Can you work these out from the model? Positions are in its coordinate system, mm. A direction names the side the tool comes from. Give positions to 0.01 mm unless a question says otherwise; leave off trailing zeros. Loops run counter-clockwise (first coordinate to the right, second up) from the corner with the lowest first, then second, coordinate; pieces in that order, holes last. Notation, with made-up numbers: (-16, 28.5) -> (0, 28.5) arc R19 cw to (0, 64.5) -> close; hole circle Ø10 at (11.5, 73.5). An arc over 180 degrees is marked (long way). One line per question, with ' | ' between items.
from build123d import *

# Parameters (mm, degrees)
SKETCH1_W               = 117.475
SKETCH1_H               = 4.7625
BOSS_EXTRUDE1_DEPTH     = 50.8
F_1_2_HOLES_DEPTH       = 78.803697293
SKETCH7_W               = 170.933784369
SKETCH7_H               = 70.3072
BOSS_EXTRUDE2_DEPTH     = 164.9349
CUT_EXTRUDE1_DEPTH      = 252.384886958
CUT_EXTRUDE1_DEPTH_BACK = 252.384886958
CUT_EXTRUDE3_DEPTH      = 208.174206511
CUT_EXTRUDE3_DEPTH_BACK = 208.174206511
SKETCH9_OUTSIDE_W       = 162.248
SKETCH9_OUTSIDE_H       = 251.148
BOSS_EXTRUDE3_DEPTH     = 7.9375
SKETCH11_OUTSIDE_W      = 1143.154
SKETCH11_OUTSIDE_H      = 1135.216
SKETCH11_OUTSIDE_R      = 11.1125
CUT_EXTRUDE4_DEPTH      = 255.208337191
CUT_EXTRUDE4_DRAFT      = -60
SKETCH12_R              = 10.795
BOSS_EXTRUDE4_DEPTH     = 64.77
SKETCH13_R              = 298.45
CUT_EXTRUDE5_DEPTH      = 254


with BuildPart() as part:
    # Sketch1 → Boss-Extrude1 (new, symmetric)
    with BuildSketch(Plane.XY):
        with Locations((0, -2.38125)):
            Rectangle(SKETCH1_W, SKETCH1_H)
    extrude(amount=BOSS_EXTRUDE1_DEPTH, both=True)

    # Sketch2 → 1-2 holes (cut, through all)
    with BuildSketch(Plane(origin=(0, 0, 0), x_dir=(1, 0, 0), z_dir=(0, 1, 0))):
        with BuildLine():
            Line((-35.649713965, 34.016189941), (-43.587213965, 29.253689941))
            ThreePointArc((-43.587213965, 29.253689941), (-50.121310059, 30.887213965), (-48.487786035, 37.421310059))
            Line((-48.487786035, 37.421310059), (-40.550286035, 42.183810059))
            ThreePointArc((-40.550286035, 42.183810059), (-34.016189941, 40.550286035), (-35.649713965, 34.016189941))
        make_face()
        with BuildLine():
            Line((-35.649713965, -34.016189941), (-43.587213965, -29.253689941))
            ThreePointArc((-43.587213965, -29.253689941), (-50.121310059, -30.887213965), (-48.487786035, -37.421310059))
            Line((-48.487786035, -37.421310059), (-40.550286035, -42.183810059))
            ThreePointArc((-40.550286035, -42.183810059), (-34.016189941, -40.550286035), (-35.649713965, -34.016189941))
        make_face()
        with BuildLine():
            Line((35.649713965, 34.016189941), (43.587213965, 29.253689941))
            ThreePointArc((43.587213965, 29.253689941), (50.121310059, 30.887213965), (48.487786035, 37.421310059))
            Line((48.487786035, 37.421310059), (40.550286035, 42.183810059))
            ThreePointArc((40.550286035, 42.183810059), (34.016189941, 40.550286035), (35.649713965, 34.016189941))
        make_face()
        with BuildLine():
            Line((35.649713965, -34.016189941), (43.587213965, -29.253689941))
            ThreePointArc((43.587213965, -29.253689941), (50.121310059, -30.887213965), (48.487786035, -37.421310059))
            Line((48.487786035, -37.421310059), (40.550286035, -42.183810059))
            ThreePointArc((40.550286035, -42.183810059), (34.016189941, -40.550286035), (35.649713965, -34.016189941))
        make_face()
    extrude(amount=-F_1_2_HOLES_DEPTH, mode=Mode.SUBTRACT)


with BuildPart() as body_2:
    # Sketch4 → Revolve1 (revolve)
    with BuildSketch(Plane.XY, mode=Mode.PRIVATE) as revolve1_sk:
        Polygon((0, -25.5651), (43.18, -25.5651), (43.18, -14.4526), (40.64, -14.4526), (40.64, -11.9126), (44.45, -11.9126), (44.45, -4.7625), (0, -4.7625), align=None)
    revolve(revolve1_sk.sketch.rotate(Axis((0, -4.7625, 0), (0, -1, 0)), 180), axis=Axis((0, -4.7625, 0), (0, -1, 0)))


with BuildPart() as body_3:
    # Sketch6 → Revolve2 (revolve)
    with BuildSketch(Plane(origin=(-63.5, 0, 0), x_dir=(0, 0, -1), z_dir=(1, 0, 0)), mode=Mode.PRIVATE) as revolve2_sk:
        with BuildLine():
            Line((-25.4, -68.58), (-25.4, -47.336363636))
            ThreePointArc((-25.4, -47.336363636), (-22.694731724, -40.805268276), (-16.163636364, -38.1))
            Line((-16.163636364, -38.1), (-14.143181818, -38.1))
            Line((-14.143181818, -38.1), (-14.143181818, -40.48125))
            Line((-14.143181818, -40.48125), (-10.102272727, -40.48125))
            Line((-10.102272727, -40.48125), (-10.102272727, -38.1))
            Line((-10.102272727, -38.1), (-6.061363636, -38.1))
            Line((-6.061363636, -38.1), (-6.061363636, -40.48125))
            Line((-6.061363636, -40.48125), (-2.020454545, -40.48125))
            Line((-2.020454545, -40.48125), (-2.020454545, -38.1))
            Line((-2.020454545, -38.1), (2.020454545, -38.1))
            Line((2.020454545, -38.1), (2.020454545, -40.48125))
            Line((2.020454545, -40.48125), (6.061363636, -40.48125))
            Line((6.061363636, -40.48125), (6.061363636, -38.1))
            Line((6.061363636, -38.1), (10.102272727, -38.1))
            Line((10.102272727, -38.1), (10.102272727, -40.48125))
            Line((10.102272727, -40.48125), (14.143181818, -40.48125))
            Line((14.143181818, -40.48125), (14.143181818, -38.1))
            Line((14.143181818, -38.1), (16.163636364, -38.1))
            ThreePointArc((16.163636364, -38.1), (22.694731724, -40.805268276), (25.4, -47.336363636))
            Line((25.4, -47.336363636), (25.4, -68.58))
            Line((25.4, -68.58), (26.67, -68.58))
            Line((26.67, -68.58), (26.67, -71.12))
            Line((26.67, -71.12), (23.495, -71.12))
            ThreePointArc((23.495, -71.12), (19.004871939, -72.979871939), (17.145, -77.47))
            ThreePointArc((17.145, -77.47), (15.476711089, -81.759997818), (11.348438966, -83.795836333))
            Line((11.348438966, -83.795836333), (5.438280517, -84.312908197))
            ThreePointArc((5.438280517, -84.312908197), (3.374144456, -85.330827454), (2.54, -87.475826363))
            Line((2.54, -87.475826363), (2.54, -93.6625))
            Line((2.54, -93.6625), (26.67, -93.6625))
            Line((26.67, -93.6625), (29.845, -93.6625))
            Line((29.845, -93.6625), (29.845, -114.3))
            Line((29.845, -114.3), (-29.845, -114.3))
            Line((-29.845, -114.3), (-29.845, -93.6625))
            Line((-29.845, -93.6625), (-26.67, -93.6625))
            Line((-26.67, -93.6625), (-2.54, -93.6625))
            Line((-2.54, -93.6625), (-2.54, -87.475826363))
            ThreePointArc((-2.54, -87.475826363), (-3.374144456, -85.330827454), (-5.438280517, -84.312908197))
            Line((-5.438280517, -84.312908197), (-11.348438966, -83.795836333))
            ThreePointArc((-11.348438966, -83.795836333), (-15.476711089, -81.759997818), (-17.145, -77.47))
            ThreePointArc((-17.145, -77.47), (-19.004871939, -72.979871939), (-23.495, -71.12))
            Line((-23.495, -71.12), (-26.67, -71.12))
            Line((-26.67, -71.12), (-26.67, -68.58))
            Line((-26.67, -68.58), (-25.4, -68.58))
        make_face()
    revolve(revolve2_sk.sketch.rotate(Axis((-63.5, -114.3, 111.145303652), (0, 0, -1)), 90), axis=Axis((-63.5, -114.3, 111.145303652), (0, 0, -1)))


with BuildPart() as body_4:
    # Sketch7 → Boss-Extrude2 (new body)
    with BuildSketch(Plane.XZ.offset(25.5651)):
        with Locations((-54.233107816, 0)):
            Rectangle(SKETCH7_W, SKETCH7_H)
    extrude(amount=BOSS_EXTRUDE2_DEPTH)

    # Sketch8 → Cut-Extrude1 (cut, two sides: drawn at the far end of the back side and taken through both)
    with BuildSketch(Plane.XY.offset(35.1536).offset(-CUT_EXTRUDE1_DEPTH_BACK)):
        with BuildLine():
            Line((313.51958325, 368.901075357), (31.233784369, -25.5651))
            Line((31.233784369, -25.5651), (-42.844161681, -129.081621811))
            ThreePointArc((-42.844161681, -129.081621811), (-78.281621811, -134.955838319), (-84.155838319, -99.518378189))
            Line((-84.155838319, -99.518378189), (-31.233784369, -25.5651))
            Line((-31.233784369, -25.5651), (251.052014512, 368.901075357))
            Line((251.052014512, 368.901075357), (251.052014512, -601.230535819))
            Line((251.052014512, -601.230535819), (313.51958325, -601.230535819))
            Line((313.51958325, -601.230535819), (313.51958325, 368.901075357))
        make_face()
    extrude(amount=CUT_EXTRUDE1_DEPTH + CUT_EXTRUDE1_DEPTH_BACK, mode=Mode.SUBTRACT)

    # Sketch9 outside → Cut-Extrude3 (cut, two sides: drawn at the far end of the back side and taken through both)
    with BuildSketch(Plane(origin=(0, -144.306693689, 0), x_dir=(0, 0, -1), z_dir=(-1, 0, 0)).offset(-CUT_EXTRUDE3_DEPTH_BACK)):
        with Locations((0, -49.057)):
            Rectangle(SKETCH9_OUTSIDE_W, SKETCH9_OUTSIDE_H)
        Polygon((35.1536, 46.193306311), (35.1536, -106.206693689), (29.815484467, -118.741593689), (27.046884467, -118.741593689), (32.385, -106.206693689), (32.385, 46.193306311), align=None, mode=Mode.SUBTRACT)
        Polygon((-27.046884467, -118.741593689), (-29.815484467, -118.741593689), (-35.1536, -106.206693689), (-35.1536, 46.193306311), (-32.385, 46.193306311), (-32.385, -106.206693689), align=None, mode=Mode.SUBTRACT)
    extrude(amount=CUT_EXTRUDE3_DEPTH + CUT_EXTRUDE3_DEPTH_BACK, mode=Mode.SUBTRACT)


with BuildPart() as cut_extrude3_piece_1:
    # of the separate pieces the step leaves, piece 1, a body of its own (cut_extrude3_pieces)
    add(body_4.part.solids().sort_by_distance((31.233784369, -25.5651, -29.815484467))[0])



with BuildPart() as cut_extrude3_piece_2:
    # of the separate pieces the step leaves, piece 2, a body of its own (cut_extrude3_pieces)
    add(body_4.part.solids().sort_by_distance((22.263625502, -38.1, 35.1536))[0])


with BuildPart() as body_6:
    # Sketch10 → Boss-Extrude3 (new body)
    with BuildSketch(Plane.XY.offset(35.1536)):
        Polygon((-63.5, -101.468390267), (-74.6125, -107.884195134), (-74.6125, -120.715804866), (-63.5, -127.131609733), (-52.3875, -120.715804866), (-52.3875, -107.884195134), align=None)
    extrude(amount=BOSS_EXTRUDE3_DEPTH)


with BuildPart() as cut_extrude4_tool:
    # Sketch11 outside → Cut-Extrude4 (with draft: the straight prism first)
    with BuildSketch(Plane.XY.offset(43.0911)):
        with Locations((-40.481, -95.25)):
            Rectangle(SKETCH11_OUTSIDE_W, SKETCH11_OUTSIDE_H)
        with Locations((-63.5, -114.3)):
            Circle(SKETCH11_OUTSIDE_R, mode=Mode.SUBTRACT)
    extrude(amount=-CUT_EXTRUDE4_DEPTH)
    # Cut-Extrude4: the draft: its side faces are tilted about the plane it starts from
    cut_extrude4_sides = [cut_extrude4_tool.faces().sort_by_distance(p)[0] for p in [
        (-40.481, -662.858, -84.513068595),
        (531.096, -95.25, -84.513068595),
        (-40.481, 472.358, -84.513068595),
        (-612.058, -95.25, -84.513068595),
        (-74.6125, -114.3, -84.513068595),
    ]]
    draft(cut_extrude4_sides, Plane.XY.offset(43.0911), CUT_EXTRUDE4_DRAFT)


with BuildPart() as body_6_1:
    add(body_6.part)

    # Cut-Extrude4: cut by cut_extrude4_tool
    add(cut_extrude4_tool.part, mode=Mode.SUBTRACT)


with BuildPart() as body_7:
    # Mirror1: mirrored copy
    add(body_6_1.part.mirror(Plane.XY))


with BuildPart() as cut_extrude3_piece_1_1:
    add(cut_extrude3_piece_1.part)

    add(cut_extrude3_piece_2.part)  # Boss-Extrude4 merges Cut-Extrude3 piece 2
    # Sketch12 → Boss-Extrude4 (add)
    with BuildSketch(Plane.XY.offset(-32.385)):
        with Locations(Location((-63.5, -114.3, 0), (0, 0, 180))):
            Circle(SKETCH12_R)
    extrude(amount=BOSS_EXTRUDE4_DEPTH)

    # Combine1: union body 7, body 6, body 2, part
    add(body_7.part)
    add(body_6_1.part)
    add(body_2.part)
    add(part.part)


with BuildPart() as cut_extrude5_tool:
    # Sketch13 → Cut-Extrude5 (new body)
    with BuildSketch(Plane.XZ.offset(11.9126)):
        Circle(SKETCH13_R)
    extrude(amount=CUT_EXTRUDE5_DEPTH)


with BuildPart() as body_3_1:
    add(body_3.part)

    # Cut-Extrude5: cut by cut_extrude5_tool
    add(cut_extrude5_tool.part, mode=Mode.SUBTRACT)


with BuildPart() as cut_extrude3_piece_1_2:
    add(cut_extrude3_piece_1_1.part)

    # Cut-Extrude5: cut by cut_extrude5_tool
    add(cut_extrude5_tool.part, mode=Mode.SUBTRACT)


solid = cut_extrude3_piece_1_2.part
Q1. On a 3-axis mill with a long thin cutter (end or side, diameter ignored), from which of +Z, -Z, +X, -X, +Y, -Y can I reach the whole of each face in a straight line? I mean faces 1 (the face through (-1, 0, 1)), 2 (the face through (44.57, -2.35, 39.77)), 3 (the face through (-40, -4.762, 23)). Say none if no direction works.
Entries:
face 1: +Z, -Z, +X, -X, +Y | face 2: +Y, -Y | face 3: -Y
Q2. If we section it at B-B (z = 0): Write out the boundary of the cut face in (x, y), plus the area to 3 significant figures.
Entries:
outline: (-58.74, -4.76) -> (-44.45, -4.76) -> (-44.45, -11.91) -> (44.45, -11.91) -> (44.45, -4.76) -> (58.74, -4.76) -> (58.74, 0) -> (-58.74, 0) -> close | area: 1,200 mm²
Q3. For pin 1 Ø3 at (y, z) = (-10, -13.5) entering from +X; pin 2 Ø1 at (x, z) = (-28, -17) entering from +Y; pin 3 Ø3 at (x, y) = (-32.5, -9.5) entering from +Z; pin 4 Ø4 at (y, z) = (-9, -40) entering from -X, each with a flat end and sliding along its axis, tell me the tip position at first contact or that it passes through.
Entries:
pin 1: x = 42.8 | pin 2: y = 0 | pin 3: z = 31.86 | pin 4: x = -23.06
Q4. If we section it at A-A (y = -2.5): Write out the boundary of the cut face in (x, z) (1 decimal), plus the area to 3 significant figures.
Entries:
outline: (-58.7, -50.8) -> (58.7, -50.8) -> (58.7, 50.8) -> (-58.7, 50.8) -> close; hole (-48.5, -37.4) -> (-40.6, -42.2) arc R4.8 ccw to (-35.6, -34) -> (-43.6, -29.3) arc R4.8 ccw to start; hole (-48.5, 37.4) arc R4.8 ccw to (-43.6, 29.3) -> (-35.6, 34) arc R4.8 ccw to (-40.6, 42.2) -> close; hole (35.6, -34) arc R4.8 ccw to (40.6, -42.2) -> (48.5, -37.4) arc R4.8 ccw to (43.6, -29.3) -> close; hole (35.6, 34) -> (43.6, 29.3) arc R4.8 ccw to (48.5, 37.4) -> (40.6, 42.2) arc R4.8 ccw to start | area: 11,300 mm²
Q5. If we mould it in two halves opening along X, with no side actions, what happens to faces 4 (the face through (-1, -2, 50.8)), 5 (the face through (-58.738, -2, 1)), 6 (the face through (-34.07, -2.35, 40.64)), 7 (the face through (58.738, -2, 1))? For each: pulls with the +X half, pulls with the -X half, needs draft (parallel to the pull), parting line crosses it, or undercut.
Entries:
face 4: needs draft | face 5: pulls with the -X half | face 6: undercut | face 7: pulls with the +X half
Q6. If I drill on probe 1 along Z at (x, y) = (49, -2); probe 2 along X at (y, z) = (-7, -1.5); probe 3 along X at (y, z) = (-5, -24), over which ranges is the centre line in solid material (lowest first)? Write a range as from..to.
Entries:
probe 1: -50.8..-37.07, -29.61..29.61, 37.07..50.8 | probe 2: -44.42..44.42 | probe 3: -37.41..37.41
Q7. If we section it at C-C (x = 0): Write out the boundary of the cut face in (y, z).
Entries:
outline: (-11.91, -44.45) -> (-4.76, -44.45) -> (-4.76, -50.8) -> (0, -50.8) -> (0, 50.8) -> (-4.76, 50.8) -> (-4.76, 44.45) -> (-11.91, 44.45) -> close
Q8. If we section it at D-D (x = 38.1): Write out the boundary of the cut face in (y, z), plus the area to 3 significant figures.
Entries:
outline: (-11.91, -22.9) -> (-4.76, -22.9) -> (-4.76, -32.55) -> (0, -32.55) -> (0, 32.55) -> (-4.76, 32.55) -> (-4.76, 22.9) -> (-11.91, 22.9) -> close; (-4.76, -50.8) -> (0, -50.8) -> (0, -42.86) -> (-4.76, -42.86) -> close; (-4.76, 42.86) -> (0, 42.86) -> (0, 50.8) -> (-4.76, 50.8) -> close | area: 713 mm²
